Read the model definition and answer for the solid it produces. Units are mm, in the model's axes. A direction names the side the tool comes from. Give positions to 0.01 mm unless a question says otherwise; leave off trailing zeros. Loops run counter-clockwise (first coordinate to the right, second up) from the corner with the lowest first, then second, coordinate; pieces in that order, holes last. Notation, with made-up numbers: (88, -24) - (124, -24) arc R18 ccw to (124, -7) - close; hole circle Ø5 at (21, -2.5). An arc over 180 degrees is marked (long way). Write each question's results on one line, items separated by ' | '. Start each with the question number.
Q1. Given pin 1 (4.5 mm diameter, centred on y = -20, z = -75.2, fed in from -X); pin 2 (3.5 mm diameter, centred on y = -20, z = -82.7, fed in from +X); pin 3 (4.5 mm diameter, centred on x = 1, y = -4.5, fed in from -Z); pin 4 (8 mm diameter, centred on x = -10, z = -77.5, fed in from -Y), each flat-ended and moving along its own axis, determine where each tip first touches the part or whether it passes through.
Q2. The part is cut by section D-D, the plane z = -71.75. Write down the section's boundary in (x, y), plus the area to 3 significant figures.
Q3. The part is cut by section A-A, the plane y = -20. Write down the section's boundary in (x, z), plus the area to 3 significant figures.
Q4. The part is cut by section C-C, the plane y = -10. Write down the section's boundary in (x, z), plus the area to 3 significant figures.
Q5. Find the intervals of material crossed by line 1 (Z direction, x = 58.5, y = -20); line 2 (Z direction, x = 67.55, y = -10); line 3 (Y direction, x = 43, z = -88.25), in increasing order. Write a range as from..to.
Q6. The part is cut by section B-B, the plane z = -89. Write down the section's boundary in (x, y).
Q7. For faces 1 (the flat face through (61, -25, -83)), 2 (the flat face through (35, -10, -70.198)), 3 (the flat face through (65.386, -20, -83)), 4 (the flat face through (51.386, -20, -83)), 5 (the flat face through (11.386, -7, -92)), determine the directions among +Z, -Z, +X, -X, +Y, -Y from which every point of the face is accessible in a straight line to the end or side of a thin tool.
Q8. Determine the mould class of faces 6 (the flat face through (49, -10, -95.198)), 7 (the flat face through (26, 0, -83)), 8 (the flat face through (65.386, -10, -83)) for opening direction Z: +Z half, -Z half, draft (parallel to the pull), parting line (faces both ways), or undercut.
```python
from build123d import *

# Parameters (mm, degrees)
F0_W     = 6
F0_H     = 2
F0_W_2   = 3.464102
F0_H_2   = 20
F0_W_3   = 20
F0_H_3   = 5
F1_DEPTH = 25
F3_DEPTH = 25.001
F4_R     = 2.5
F5_DEPTH = 20.001
F6_R     = 2
F7_DEPTH = 6
F8_SIZE2 = 1.154341
F8_SIZE  = 5


with BuildPart() as f1:
    # F0 (on Front) → F1 (new body)
    with BuildSketch(Plane.XZ):
        with Locations((68.386151, -81.697741)):
            Rectangle(F0_W, F0_H)
        with Locations((68.386151, -83.697741)):
            Rectangle(F0_W, F0_H)
        Polygon((51.386151, -75.197741), (51.386151, -70.197741), (-20.149747, -70.197741), (-20.149747, -90.197741), (11.386151, -90.197741), (11.386151, -93.197741), (14.850253, -95.197741), (51.386151, -95.197741), (51.386151, -90.197741), align=None)
        with Locations((-21.881798, -80.197741)):
            Rectangle(F0_W_2, F0_H_2)
        with Locations((61.386151, -72.697741)):
            Rectangle(F0_W_3, F0_H_3)
        with Locations((61.386151, -92.697741)):
            Rectangle(F0_W_3, F0_H_3)
        Polygon((71.386151, -80.697741), (71.386151, -75.197741), (51.386151, -75.197741), (51.386151, -90.197741), (71.386151, -90.197741), (71.386151, -84.697741), (65.386151, -84.697741), (64.231451, -82.697741), (65.386151, -80.697741), align=None)
        Polygon((65.386151, -82.697741), (65.386151, -80.697741), (64.231451, -82.697741), align=None)
        Polygon((65.386151, -84.697741), (65.386151, -82.697741), (64.231451, -82.697741), align=None)
    extrude(amount=F1_DEPTH)

    # F2 (on face) → F3 (cut, through all)
    with BuildSketch(Plane.XY.offset(-70.197741)):
        Polygon((-23.613849, -25), (51.386151, -25), (51.386151, -20), (51.386151, -15), (11.386151, -15), (-23.613849, -15), align=None)
    extrude(amount=-F3_DEPTH, mode=Mode.SUBTRACT)

    # F4 (on face) → F5 (cut, through all)
    with BuildSketch(Plane(origin=(51.386151, 0, 0), x_dir=(0, -1, 0), z_dir=(-1, 0, 0))):
        with Locations((20, -75.197741)):
            Circle(F4_R)
        with Locations((20, -90.197741)):
            Circle(F4_R)
    extrude(amount=-F5_DEPTH, mode=Mode.SUBTRACT)

    # F6 (on face) → F7 (cut)
    with BuildSketch(Plane.YZ.offset(71.386151)):
        with Locations((-20, -82.697741)):
            Circle(F6_R)
        with Locations((-10, -82.697741)):
            Circle(F6_R)
    extrude(amount=-F7_DEPTH, mode=Mode.SUBTRACT)

    # F8
    f8_edges = [f1.edges().sort_by_distance(p)[0] for p in [
        (-23.613849, 0, -80.197741),
    ]]
    chamfer(f8_edges, length=F8_SIZE, length2=F8_SIZE2)


solid = f1.part
```
Check sheet entries:
1) pin 1: passes through | pin 2: stops at x = 65.39 | pin 3: stops at z = -90.2 | pin 4: stops at y = -15
2) outline: (-23.61, -15) - (51.39, -15) - (51.39, -25) - (71.39, -25) - (71.39, 0) - (-18.61, 0) - (-23.61, -1.15) - close | area: 1,620 mm^2
3) outline: (51.39, -95.2) - (71.39, -95.2) - (71.39, -92.7) - (51.39, -92.7) - close; (51.39, -87.7) - (71.39, -87.7) - (71.39, -84.7) - (65.39, -84.7) - (65.39, -80.7) - (71.39, -80.7) - (71.39, -77.7) - (51.39, -77.7) - close; (51.39, -72.7) - (71.39, -72.7) - (71.39, -70.2) - (51.39, -70.2) - close | area: 276 mm^2
4) outline: (-23.61, -90.2) - (11.39, -90.2) - (11.39, -93.2) - (14.85, -95.2) - (71.39, -95.2) - (71.39, -84.7) - (65.39, -84.7) - (65.39, -80.7) - (71.39, -80.7) - (71.39, -70.2) - (-23.61, -70.2) - close | area: 2,170 mm^2
5) line 1: z = -95.2..-92.7, -87.7..-77.7, -72.7..-70.2 | line 2: z = -95.2..-84.7, -80.7..-70.2 | line 3: y = -15..0
6) outline: (-23.61, -15) - (51.39, -15) - (51.39, -17.81) - (71.39, -17.81) - (71.39, 0) - (-18.61, 0) - (-23.61, -1.15) - close; (51.39, -25) - (71.39, -25) - (71.39, -22.19) - (51.39, -22.19) - close
7) face 1: +Z, -Z, +X, -X, -Y | face 2: +Z, +X, -X, +Y, -Y | face 3: +X | face 4: +Z, -Z, -X, -Y | face 5: -Z, -X, +Y, -Y
8) face 6: -Z half | face 7: draft | face 8: undercut
